Design review of the part built by this model. Coordinates are the model's own, in mm. Face numbers are marked on the shaded views. A direction names the side the tool comes from. Coordinates: 2 decimals unless noted, no trailing zeros. Write each loop counter-clockwise with the first axis right and the second up, starting at its lowest first coordinate (ties: lowest second). Pieces come first, ordered by that corner, then holes.
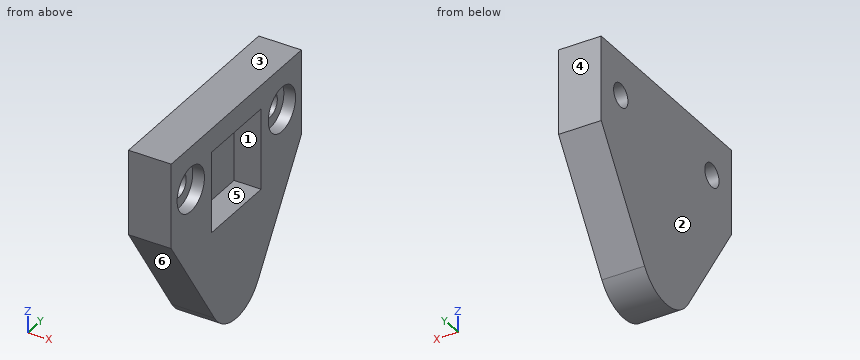
```python
from build123d import *

# Parameters (mm, degrees)
SKETCH1_W                       = 20
SKETCH1_H                       = 50
BOSS_EXTRUDE1_DEPTH             = 10
CBORE_FOR_M5_SBHCS1_D           = 5.5
CBORE_FOR_M5_SBHCS1_CBORE_D     = 10.5
CBORE_FOR_M5_SBHCS1_CBORE_DEPTH = 2.75
SKETCH5_W                       = 19.05
SKETCH5_H                       = 19.05
CUT_EXTRUDE1_DEPTH              = 6.35


with BuildPart() as part:
    # Sketch1 → Boss-Extrude1 (new body)
    with BuildSketch(Plane(origin=(0, 0, 0), x_dir=(0, 0, -1), z_dir=(1, 0, 0))):
        with Locations((-10, 0)):
            Rectangle(SKETCH1_W, SKETCH1_H)
        with BuildLine():
            ThreePointArc((25.466783574, 8.373426859), (30, 0), (25.466783574, -8.373426859))
            Line((25.466783574, -8.373426859), (0, -25))
            Line((0, -25), (0, 25))
            Line((0, 25), (25.466783574, 8.373426859))
        make_face()
    extrude(amount=BOSS_EXTRUDE1_DEPTH)

    # CBORE for M5 SBHCS1 (through all)
    with Locations(Plane(origin=(10, 0, 0), x_dir=(0, 0, -1), z_dir=(1, 0, 0))):
        with Locations((-10, 17.5), (-10, -17.5)):
            CounterBoreHole(CBORE_FOR_M5_SBHCS1_D / 2, CBORE_FOR_M5_SBHCS1_CBORE_D / 2, CBORE_FOR_M5_SBHCS1_CBORE_DEPTH)

    # Sketch5 → Cut-Extrude1 (cut)
    with BuildSketch(Plane(origin=(10, 0, 0), x_dir=(0, 0, -1), z_dir=(1, 0, 0))):
        with Locations((-4.915565879, 0)):
            Rectangle(SKETCH5_W, SKETCH5_H)
    extrude(amount=-CUT_EXTRUDE1_DEPTH, mode=Mode.SUBTRACT)


solid = part.part
```
(1) Consider section B-B (z = 10). Give the boundary of the cut face in (x, y) (3 decimals), plus the area to 3 significant figures.
(2) Consider section D-D (z = 3). Give the boundary of the cut face in (x, y) (3 decimals).
(3) Consider section A-A (x = 4.75). Give the boundary of the cut face in (y, z) (3 decimals).
(4) Mouldability with a two-part tool opening along Z and no side actions: class the marked faces 3, 4, 5 and 6 as +Z half, -Z half, draft (parallel to the pull), parting line (faces both ways), or undercut.
(5) Insertion check: pin 1 Ø9 at (y, z) = (-17.5, 10) entering from +X; pin 2 Ø5 at (x, y) = (6, 9) entering from -Z; pin 3 Ø3 at (y, z) = (-18.5, 10) entering from +X; pin 4 Ø5.5 at (y, z) = (3, 7.5) entering from +X. Each pin has a flat end and moves straight along its axis. Give the tip position at first contact, or say it passes through.
(6) For the marked faces 1 and 2, list the 3-axis set-ups (+Z, -Z, +X, -X, +Y, -Y) from which the entire face can be reached by the end or side of a thin tool; tool diameter is ignored.
(7) Consider section C-C (y = 16). Give the boundary of the cut face in (x, z), plus the area to 3 significant figures.
(8) Wall thickness on line 1 (Y direction, x = 8.1, z = 10) (3 decimals); line 2 (Y direction, x = 3.5, z = 10); line 3 (Y direction, x = 6.5, z = 3.5) (3 decimals): over which ranges is each line inside the solid? List them lowest first.
Results:
1. outline: (0, -25) - (10, -25) - (10, -22.75) - (7.25, -22.75) - (7.25, -20.25) - (0, -20.25) - close; (0, -14.75) - (7.25, -14.75) - (7.25, -12.25) - (10, -12.25) - (10, -9.525) - (3.65, -9.525) - (3.65, 9.525) - (10, 9.525) - (10, 12.25) - (7.25, 12.25) - (7.25, 14.75) - (0, 14.75) - close; (0, 20.25) - (7.25, 20.25) - (7.25, 22.75) - (10, 22.75) - (10, 25) - (0, 25) - close
1. area: 242 mm2
2. outline: (0, -25) - (10, -25) - (10, -9.525) - (3.65, -9.525) - (3.65, 9.525) - (10, 9.525) - (10, 25) - (0, 25) - close
3. outline: (-25, 0) - (-8.373, -25.467) arc R10 ccw to (8.373, -25.467) - (25, 0) - (25, 20) - (-25, 20) - close; hole circle Ø5.5 at (-17.5, 10); hole (-9.525, -4.609) - (9.525, -4.609) - (9.525, 14.441) - (-9.525, 14.441) - close; hole circle Ø5.5 at (17.5, 10)
4. face 3: +Z half
4. face 4: draft
4. face 5: undercut
4. face 6: -Z half
5. pin 1: stops at x = 7.25
5. pin 2: stops at z = -27.6
5. pin 3: passes through
5. pin 4: stops at x = 3.65
6. face 1: +X
6. face 2: +Z, -Z, -X, +Y, -Y
7. outline: (0, -13.79) - (10, -13.79) - (10, 4.97) - (7.25, 4.97) - (7.25, 7.7) - (0, 7.7) - close; (0, 12.3) - (7.25, 12.3) - (7.25, 15.03) - (10, 15.03) - (10, 20) - (0, 20) - close
7. area: 277 mm2
8. line 1: y = -25 to -22.75, -12.25 to -9.525, 9.525 to 12.25, 22.75 to 25
8. line 2: y = -25 to -20.25, -14.75 to 14.75, 20.25 to 25
8. line 3: y = -25 to -9.525, 9.525 to 25
